Can you work these out from the drawing? Everything is in mm from the part's minimum corner. A direction names the side the tool comes from. Round coordinates to 2 decimals unless told otherwise and drop trailing zeros. Write each loop counter-clockwise with the first axis right and the second up, starting at its lowest first coordinate (ties: lowest second). Pieces come first, ordered by that corner, then holes. Notation, with made-up numbers: M 11.5,79 L 26.5,79 A29 cw 26.5,112 Z; hole C -38,86 d9. An arc over 180 degrees is marked long. Use one line per item in the form item = value. Start each with the question number.
Q1. We'd pull the mould along Y, two halves only. Please class the marked faces 4, 5 and 6: +Y half, -Y half, draft (parallel to the pull), parting line (faces both ways), or undercut.
Q2. I want a section at A-A on z = 16. List the corners of the cut face in (x, y) for me.
Q3. I'm going to push flat-ended pins straight in: pin 1 Ø5 at (x, z) = (5, 16) entering from -Y; pin 2 Ø23 at (x, y) = (27.5, 30) entering from -Z; pin 3 Ø5 at (x, z) = (49, 6) entering from +Y; pin 4 Ø8 at (y, z) = (11.5, 13) entering from +X. Where does each tip first touch, or does it pass through?
Q4. I need wall thicknesses on line 1 along X through (y, z) = (3.9, 4); line 2 along Z through (x, y) = (50, 3.55); line 3 along Y through (x, z) = (28, 16.25). Which ranges of each line are inside material? Lowest first, please. Write a range as from..to.
Q5. I want a section at C-C on y = 26. List the corners of the cut face in (x, z) for me, and give its area (3 significant figures).
Q6. For the marked faces 1, 2 and 3, which set-ups out of +Z, -Z, +X, -X, +Y, -Y let a thin tool reach every point of the face, with its end or its side?
Q7. I want a section at D-D on x = 5. List the corners of the cut face in (y, z) for me, and give its area (3 significant figures).
Q8. I want a section at B-B on z = 11.5. List the corners of the cut face in (x, y) for me.
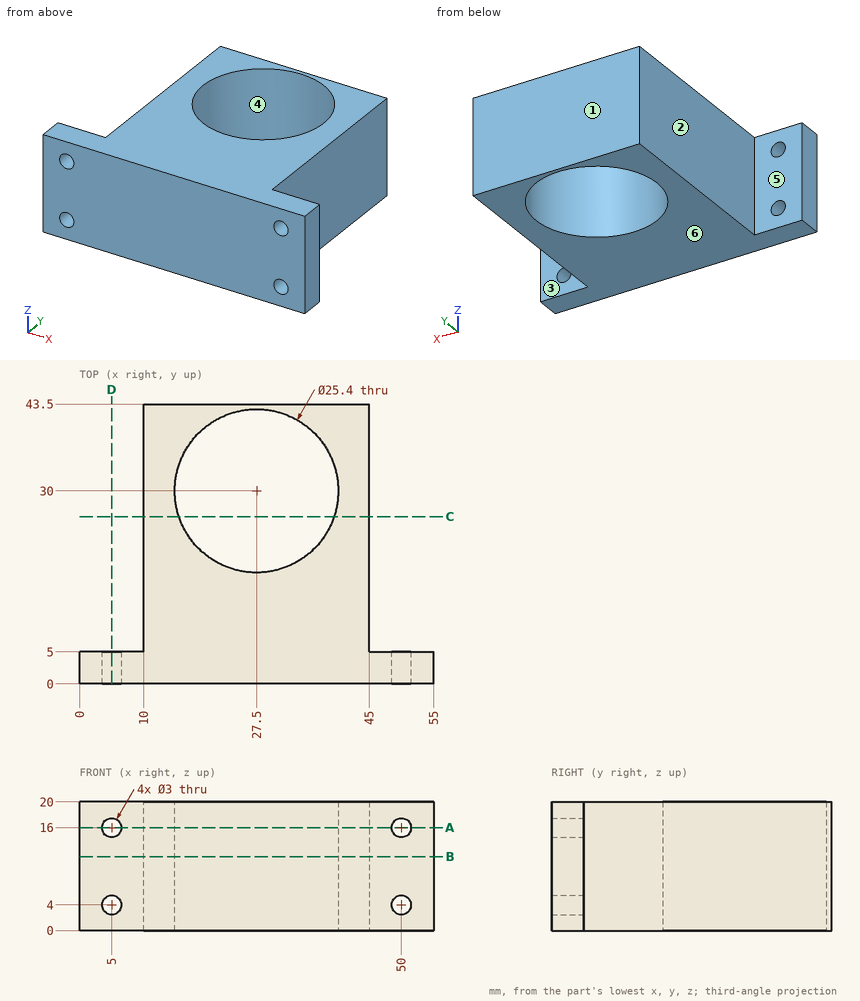
Reported:
q1.face_4 = undercut
q1.face_5 = +Y half
q1.face_6 = draft
q2.outline = M 0,0 L 3.5,0 L 3.5,5 L 0,5 Z; M 6.5,0 L 48.5,0 L 48.5,5 L 45,5 L 45,43.5 L 10,43.5 L 10,5 L 6.5,5 Z; M 51.5,0 L 55,0 L 55,5 L 51.5,5 Z; hole C 27.5,30 d25.4
q3.pin_1 = 0
q3.pin_2 = through
q3.pin_3 = 5
q3.pin_4 = 45
q4.line_1 = 0..3.5, 6.5..48.5, 51.5..55
q4.line_2 = 0..2.5, 5.5..14.5, 17.5..20
q4.line_3 = 0..17.31, 42.69..43.5
q5.outline = M 10,0 L 15.45,0 L 15.45,20 L 10,20 Z; M 39.55,0 L 45,0 L 45,20 L 39.55,20 Z
q5.area = 218 mm^2
q6.face_1 = +Z, -Z, +X, -X, +Y
q6.face_2 = +Z, -Z, -X, +Y
q6.face_3 = +Z, -Z, +X, +Y
q7.outline = M 0,0 L 5,0 L 5,2.5 L 0,2.5 Z; M 0,5.5 L 5,5.5 L 5,14.5 L 0,14.5 Z; M 0,17.5 L 5,17.5 L 5,20 L 0,20 Z
q7.area = 70.0 mm^2
q8.outline = M 0,0 L 55,0 L 55,5 L 45,5 L 45,43.5 L 10,43.5 L 10,5 L 0,5 Z; hole C 27.5,30 d25.4
